Source: CAD feature listing. Evaluate the final solid. Frame: model axes, mm. A direction names the side the tool comes from. Give positions to 0.01 mm unless a question says otherwise; leave off trailing zeros. Order: outer loops, then holes, each group sorted by start corner. A loop starts at its lowest first (then second) coordinate and runs counter-clockwise, first axis right, second up. Notation, with made-up numbers: (-12, 26.25) - (2, 26.25) arc R18 ccw to (2, 37.25) - close; hole circle Ø6 at (-7.75, 30.25). An arc over 180 degrees is marked (long way). Answer as CSV lines item,"result".
```python
from build123d import *

# Parameters (mm, degrees)
ESQUISSE1_W             = 300
ESQUISSE1_H             = 200
EXTRUSION1_DEPTH        = 350
COQUE2_T                = -5
ESQUISSE2_R             = 2
ENL_V_MAT_EXTRU_1_DEPTH = 394.700393701
CONG_1_R                = 10


with BuildPart() as part:
    # Esquisse1 → Extrusion1 (new body)
    with BuildSketch(Plane(origin=(0, 0, 0), x_dir=(1, 0, 0), z_dir=(0, 1, 0))):
        Rectangle(ESQUISSE1_W, ESQUISSE1_H)
    extrude(amount=EXTRUSION1_DEPTH)

    # Coque2
    coque2_openings = [part.faces().sort_by_distance(p)[0] for p in [
        (0, 0, 0),
    ]]
    offset(amount=COQUE2_T, openings=coque2_openings, kind=Kind.INTERSECTION)

    # Esquisse2 → Enlèv. mat.-Extru.1 (cut, through all)
    with BuildSketch(Plane(origin=(0, 350, 0), x_dir=(1, 0, 0), z_dir=(0, 1, 0))):
        with Locations(Location((-36, 36, 0), (0, 0, 270))):
            Circle(ESQUISSE2_R)
        with Locations(Location((36, 36, 0), (0, 0, 270))):
            Circle(ESQUISSE2_R)
        with Locations(Location((-36, -36, 0), (0, 0, 270))):
            Circle(ESQUISSE2_R)
        with Locations(Location((36, -36, 0), (0, 0, 270))):
            Circle(ESQUISSE2_R)
    extrude(amount=-ENL_V_MAT_EXTRU_1_DEPTH, mode=Mode.SUBTRACT)

    # Congé1
    cong_1_edges = [part.edges().sort_by_distance(p)[0] for p in [
        (150, 350, 0),
        (0, 350, -100),
        (-150, 350, 0),
        (0, 350, 100),
        (-150, 175, -100),
        (150, 175, -100),
        (150, 175, 100),
        (-150, 175, 100),
    ]]
    fillet(cong_1_edges, radius=CONG_1_R)


solid = part.part
```
(1) Cut plane C-C (x = 93). Return loops of the section in (y, z), then the cut area to 3 significant figures.
Completed:
outline,"(0, -100) - (340, -100) arc R10 ccw to (350, -90) - (350, 90) arc R10 ccw to (340, 100) - (0, 100) - (0, 95) - (345, 95) - (345, -95) - (0, -95) - close"
area,"4,410 mm²"
(2) Ray query, line 1 (Z direction, x = -20, y = 126); line 2 (X direction, y = 346.55, z = -36); line 3 (X direction, y = 348.85, z = 36). Return the intervals inside material, ascending. Write a range as from..to.
Completed:
line 1,"-100..-95, 95..100"
line 2,"-147.56..-38, -34..34, 38..147.56"
line 3,"-144.66..-38, -34..34, 38..144.66"
(3) Access query for faces 1 (the flat face through (-2, 170, -95)), 2 (the cylindrical face through (146.99, 172.38, -97.15)). Directions: +Z, -Z, +X, -X, +Y, -Y. A direction counts if a zero-diameter tool reaches every point of the face in a straight line with its end or side. Return the directions, or none.
Completed:
face 1,"-Y"
face 2,"-Z, +X, +Y, -Y"
(4) Contact query for flat-ended pins moving along their axis: pin 1 (2.5 mm diameter, centred on x = 36, z = -36, fed in from +Y); pin 2 (10 mm diameter, centred on x = 94.5, z = 68.5, fed in from -Y). Output: stop coordinate, or through.
Completed:
pin 1,"through"
pin 2,"y = 345"
(5) Cut plane B-B (z = -3). Return loops of the section in (x, y), then the cut area to 3 significant figures.
Completed:
outline,"(-150, 0) - (-145, 0) - (-145, 345) - (145, 345) - (145, 0) - (150, 0) - (150, 340) arc R10 ccw to (140, 350) - (-140, 350) arc R10 ccw to (-150, 340) - close"
area,"4,910 mm²"
(6) Cut plane A-A (y = 247). Return loops of the section in (x, z), then the cut area to 3 significant figures.
Completed:
outline,"(-150, -90) arc R10 ccw to (-140, -100) - (140, -100) arc R10 ccw to (150, -90) - (150, 90) arc R10 ccw to (140, 100) - (-140, 100) arc R10 ccw to (-150, 90) - close; hole (-145, -95) - (145, -95) - (145, 95) - (-145, 95) - close"
area,"4,810 mm²"
(7) Mould query, pull axis X, two halves, no side actions, for faces 3 (the cylindrical face through (-147.15, 172.38, 96.99)), 4 (the flat face through (-145, 170, 1)), 5 (the flat face through (-2, 350, -1)), 6 (the flat face through (-2, 345, -1)). Classes: released by +X, released by -X, zero draft, split by the parting line, or undercut.
Completed:
face 3,"released by -X"
face 4,"undercut"
face 5,"zero draft"
face 6,"undercut"
